Could you check a few things on this model? Use its own coordinates, in mm. A direction names the side the tool comes from. Round coordinates to 2 decimals unless told otherwise and drop trailing zeros. Write each loop counter-clockwise with the first axis right and the second up, starting at its lowest first coordinate (ties: lowest second). Pieces come first, ordered by that corner, then holes. Notation, with made-up numbers: (79, 45.25) -> (111, 45.25) arc R24 ccw to (111, 61.25) -> close; hole circle Ø10 at (34, -10.5). An arc over 180 degrees is marked (long way). Return JSON: item names as keys, results as strings.
from build123d import *

# Parameters (mm, degrees)
BOSS_EXTRUDE4_DEPTH = 25.4
SKETCH9_R           = 3.175
CUT_EXTRUDE3_DEPTH  = 30.48


with BuildPart() as part:
    # Sketch8 → Boss-Extrude4 (new body)
    with BuildSketch(Plane(origin=(0, 0, 0), x_dir=(1, 0, 0), z_dir=(0, 1, 0))):
        with BuildLine():
            Line((-0.905835842, 6.259395066), (-0.508, 7.800206655))
            Line((-0.508, 7.800206655), (0.508, 7.800206655))
            Line((0.508, 7.800206655), (0.905835842, 6.259395066))
            ThreePointArc((0.905835842, 6.259395066), (2.420319636, 5.843168491), (3.785538031, 5.066583363))
            Line((3.785538031, 5.066583363), (5.156368775, 5.874789265))
            Line((5.156368775, 5.874789265), (5.874789265, 5.156368775))
            Line((5.874789265, 5.156368775), (5.066583363, 3.785538031))
            ThreePointArc((5.066583363, 3.785538031), (5.843168491, 2.420319636), (6.259395066, 0.905835842))
            Line((6.259395066, 0.905835842), (7.800206655, 0.508))
            Line((7.800206655, 0.508), (7.800206655, -0.508))
            Line((7.800206655, -0.508), (6.259395066, -0.905835842))
            ThreePointArc((6.259395066, -0.905835842), (5.843168491, -2.420319636), (5.066583363, -3.785538031))
            Line((5.066583363, -3.785538031), (5.874789265, -5.156368775))
            Line((5.874789265, -5.156368775), (5.156368775, -5.874789265))
            Line((5.156368775, -5.874789265), (3.785538031, -5.066583363))
            ThreePointArc((3.785538031, -5.066583363), (2.420319636, -5.843168491), (0.905835842, -6.259395066))
            Line((0.905835842, -6.259395066), (0.508, -7.800206655))
            Line((0.508, -7.800206655), (-0.508, -7.800206655))
            Line((-0.508, -7.800206655), (-0.905835842, -6.259395066))
            ThreePointArc((-0.905835842, -6.259395066), (-2.420319636, -5.843168491), (-3.785538031, -5.066583363))
            Line((-3.785538031, -5.066583363), (-5.156368775, -5.874789265))
            Line((-5.156368775, -5.874789265), (-5.874789265, -5.156368775))
            Line((-5.874789265, -5.156368775), (-5.066583363, -3.785538031))
            ThreePointArc((-5.066583363, -3.785538031), (-5.843168491, -2.420319636), (-6.259395066, -0.905835842))
            Line((-6.259395066, -0.905835842), (-7.800206655, -0.508))
            Line((-7.800206655, -0.508), (-7.800206655, 0.508))
            Line((-7.800206655, 0.508), (-6.259395066, 0.905835842))
            ThreePointArc((-6.259395066, 0.905835842), (-5.843168491, 2.420319636), (-5.066583363, 3.785538031))
            Line((-5.066583363, 3.785538031), (-5.874789265, 5.156368775))
            Line((-5.874789265, 5.156368775), (-5.156368775, 5.874789265))
            Line((-5.156368775, 5.874789265), (-3.785538031, 5.066583363))
            ThreePointArc((-3.785538031, 5.066583363), (-2.420319636, 5.843168491), (-0.905835842, 6.259395066))
        make_face()
    extrude(amount=BOSS_EXTRUDE4_DEPTH)

    # Sketch9 → Cut-Extrude3 (cut)
    with BuildSketch(Plane(origin=(0, 25.4, 0), x_dir=(1, 0, 0), z_dir=(0, 1, 0))):
        Circle(SKETCH9_R)
    extrude(amount=-CUT_EXTRUDE3_DEPTH, mode=Mode.SUBTRACT)


solid = part.part
1) Will these pins go through, and if not, where does the flat tip stop? pin 1 Ø2 at (x, z) = (-0.5, 2.5) entering from +Y; pin 2 Ø2 at (y, z) = (21, 2) entering from +X.
Return value:
{"pin 1": "y = 25.4", "pin 2": "x = 6.25"}
2) I want a section at A-A, the plane z = 0. Please give me the cut outline in (x, y) (3 decimals).
Return value:
{"outline": "(-7.8, 0) -> (-3.175, 0) -> (-3.175, 25.4) -> (-7.8, 25.4) -> close; (3.175, 0) -> (7.8, 0) -> (7.8, 25.4) -> (3.175, 25.4) -> close"}
3) For faces 1 (the face through (6, 13, -2)), 2 (the face through (2, 13, 6)), 3 (the face through (-2, 13, -6)), 4 (the face through (-5.476, 12.522, 4.481)), which set-ups out of +Z, -Z, +X, -X, +Y, -Y let a thin tool reach every point of the face, with its end or its side?
Return value:
{"face 1": "+X, +Y, -Y", "face 2": "+Z, +Y, -Y", "face 3": "-Z, +Y, -Y", "face 4": "-X, +Y, -Y"}
4) I want a section at B-B, the plane x = 0. Please give me the cut outline in (y, z) (3 decimals).
Return value:
{"outline": "(0, -7.8) -> (25.4, -7.8) -> (25.4, -3.175) -> (0, -3.175) -> close; (0, 3.175) -> (25.4, 3.175) -> (25.4, 7.8) -> (0, 7.8) -> close"}
5) I want a section at D-D, the plane x = -4.75. Please give me the cut outline in (y, z), and give its area (3 significant figures).
Return value:
{"outline": "(0, -5.64) -> (25.4, -5.64) -> (25.4, 5.64) -> (0, 5.64) -> close", "area": "286 mm²"}
6) Thinking about a two-plate mould opening in Z: for faces 5 (the face through (-0.704, 12.522, 7.041)), 6 (the face through (-7.041, 12.522, -0.704)), 7 (the face through (-0.69, 12.88, 3.1)), 8 (the face through (7.8, 13, 0)), which applies, pulls with the +Z half, pulls with the -Z half, needs draft (parallel to the pull), parting line crosses it, or undercut?
Return value:
{"face 5": "pulls with the +Z half", "face 6": "pulls with the -Z half", "face 7": "undercut", "face 8": "needs draft"}
7) If I drill on probe 1 along Z at (x, y) = (0, 11) (3 decimals); probe 2 along Z at (x, y) = (-5.75, 15.25), over which ranges is the centre line in solid material (lowest first)? Write a range as [from, to].
Return value:
{"probe 1": "[-7.8, -3.175], [3.175, 7.8]", "probe 2": "[-5.28, -4.94], [-2.63, 2.63], [4.94, 5.28]"}
